The listing builds one solid part. Answer for the finished solid, in the listing's coordinates (mm). Face numbers are marked on the shaded views. A direction names the side the tool comes from. Round coordinates to 2 decimals unless told otherwise and drop trailing zeros. Write each loop counter-clockwise with the first axis right and the second up, starting at its lowest first coordinate (ties: lowest second). Pieces come first, ordered by that corner, then holes. Notation, with made-up numbers: (-15, 28) - (8, 28) arc R18 cw to (8, 42) - close; hole circle Ø3 at (44.5, 31). An arc over 180 degrees is marked (long way). Answer as CSV lines item,"result". Start each with the question number.
Item 1: For a pull along Y with two mould halves and no side action, classify the marked faces 1, 2, 3 and 4 as pulls with the +Y half, pulls with the -Y half, needs draft (parallel to the pull), parting line crosses it, or undercut.
Item 2: A cutting plane is placed at C-C on z = 132. Determine the outline of the cut face in (x, y), and give its area (3 significant figures).
Item 3: Which of the six approach directions +Z, -Z, +X, -X, +Y, -Y give full straight-line access (tool end or side, diameter ignored) to the marked faces 5 and 6?
Item 4: A cutting plane is placed at A-A on y = 10. Determine the outline of the cut face in (x, z), and give its area (3 significant figures).
Item 5: Straight lines are drawn through the part: line 1 along Z through (x, y) = (40, 74.5); line 2 along Z through (x, y) = (40, 86); line 3 along Y through (x, z) = (84, 42). For each, find the intervals that lie inside material, in ascending order. Write a range as [from, to].
Item 6: A cutting plane is placed at B-B on x = 44.5. Determine the outline of the cut face in (y, z), and give its area (3 significant figures).
Item 7: Flat-ended cylindrical pins translate along their axes: pin 1 (24 mm diameter, centred on x = 24, y = 32.5, fed in from -Z); pin 2 (8 mm diameter, centred on y = 63.5, z = 83.5, fed in from +X); pin 3 (8 mm diameter, centred on x = 49.5, z = 34, fed in from +Y); pin 4 (1.1 mm diameter, centred on x = 25.5, z = 81.5, fed in from +Y). Find the tip coordinate at first contact, or state that the pin passes through.
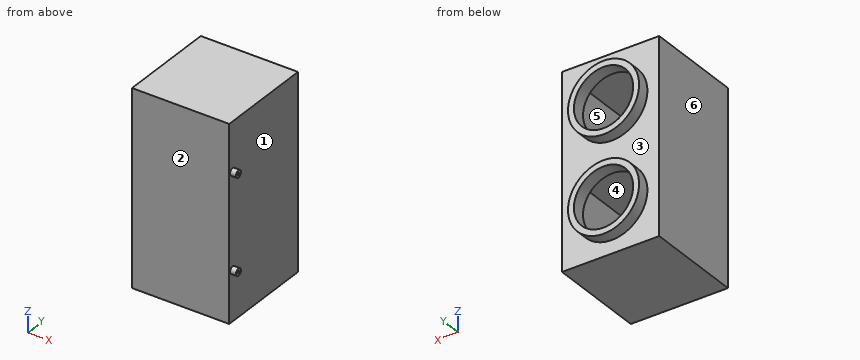
Autodesk Inventor part; units mm, degrees
ref_plane "YZ Plane" through (0, 0, 0) normal (1, 0, 0) x (0, 1, 0)
ref_plane "XZ Plane" through (0, 0, 0) normal (0, 1, 0) x (-1, 0, 0)
ref_plane "XY Plane" through (0, 0, 0) normal (0, 0, 1) x (1, 0, 0)
sketch "Sketch1" plane through (0, 0, 0) normal (0, 0, 1) x (1, 0, 0)
  line L0 (0, 0) -> (82, 0)
  line L1 (82, 0) -> (82, 82)
  line L2 (82, 82) -> (0, 82)
  line L3 (0, 82) -> (0, 0)
  dimension "d0" = 82
  dimension "d1" = 82
extrude "Extrusion1" add sketch "Sketch1" along normal blind 163
shell "Shell1" thickness 1 removed faces 1 at (54.6667, 82, 54.3333)
sketch "Sketch6" plane through (82, 0, 0) normal (1, 0, 0) x (0, 0, -1)
  circle A0 centre (-122, 4) radius 1
  circle A1 centre (-122, 4) radius 3
  line L0 (0, 0) -> (0, 82)
  line L1 (0, 0) -> (-163, 0)
  line L2 (-163, 0) -> (-163, 82)
  dimension "d18" = 2
  dimension "d19" = 2
  dimension "d21" = 4
  dimension "d50" = 41
extrude "Extrusion5" add sketch "Sketch6" along normal blind 5
thread "Thread1"
sketch "Sketch7" plane through (82, 4, 122) normal (1, 0, 0) x (0, 0, -1)
  circle A0 centre (0, 0) radius 1
  circle A1 centre (0, 0) radius 1
  point P0 (122, -4)
extrude "Extrusion6" cut sketch "Sketch7" against normal blind 5
sketch "Sketch8" plane through (0, 82, 0) normal (0, 1, 0) x (1, 0, 0)
  line L0 (0, 0) -> (0, -163)
  line L1 (82, 0) -> (82, -163)
  line L2 (0, 0) -> (82, 0)
  line L3 (82, 0) -> (82, -163)
  line L4 (82, -163) -> (0, -163)
  line L5 (0, -163) -> (0, 0)
  point P0 (0, -163)
extrude "Extrusion7" add sketch "Sketch8" along normal blind 1
sketch "Sketch9" plane through (0, 83, 0) normal (0, 1, 0) x (1, 0, 0)
  circle A0 centre (40, -122) radius 25
  circle A1 centre (40, -122) radius 30
  line L0 (0, 0) -> (0, -163)
  line L1 (0, -163) -> (82, -163)
  line L2 (1, -1) -> (1, -162)
  line L3 (1, -81.5) -> (81, -81.5)
  line L4 (81, -1) -> (81, -162)
  dimension "d30" = 50
  dimension "d31" = 40
  dimension "d32" = 41
  dimension "d33" = 5
extrude "Extrusion8" add sketch "Sketch9" along normal blind 10
sketch "Sketch10" plane through (40, 83, 122) normal (0, 1, 0) x (1, 0, 0)
  circle A0 centre (0, 0) radius 25
  point P0 (-40, 122)
extrude "Extrusion9" cut sketch "Sketch10" against normal blind 10
thread "Thread2"
sketch "Sketch12" plane through (1, 1, 1) normal (0, 1, 0) x (1, 0, 0)
  line L0 (0, 0) -> (0, -161)
  line L1 (0, -81) -> (80, -81)
  line L2 (80, -81) -> (80, -80)
  line L3 (80, -80) -> (0, -80)
  line L4 (0, -80) -> (0, -81)
  line L5 (80, 0) -> (80, -161)
  line L6 (0, -161) -> (80, -161)
  point P0 (-1, 1)
  point P1 (0, -80)
  dimension "d44" = 1
  dimension "d45" = 80
extrude "Extrusion11" add sketch "Sketch12" along normal blind 80 contours L3 L2 L1 L0
sketch "Sketch3" plane through (1, 82, 1) normal (0, 0, 1) x (1, 0, 0)
  line L0 (0, -81) -> (80, -81)
  line L1 (80, -81) -> (0, -78)
  line L2 (0, -78) -> (0, -81)
  point P0 (-1, -82)
  dimension "d5" = 3
extrude "Extrusion12" add sketch "Sketch3" along normal up to surface (161 mm away)
pattern_linear "Rectangular Pattern1" count 2 spacing 81 along (0, 0, -1) of "Extrusion8", "Extrusion9"
pattern_linear "Rectangular Pattern3" count 2 spacing 80 along (0, 0, -1) of "Extrusion5", "Extrusion6"
properties part number "BoxChem"
Geometry says:
1,face 1,"needs draft"
1,face 2,"pulls with the -Y half"
1,face 3,"pulls with the +Y half"
1,face 4,"undercut"
2,outline,"(0, 0) - (82, 0) - (82, 83) - (68.28, 83) - (68.28, 93) - (62.91, 93) - (62.91, 82) - (81, 82) - (81, 1) - (1, 4) - (1, 82) - (17.09, 82) - (17.09, 93) - (11.72, 93) - (11.72, 83) - (0, 83) - close"
2,area,"508 mm^2"
3,face 5,"none"
3,face 6,"+Z, -Z, -X, +Y, -Y"
4,outline,"(0, 0) - (82, 0) - (82, 163) - (0, 163) - close; hole (1, 1) - (81, 1) - (81, 81) - (1, 81) - close; hole (1, 82) - (81, 82) - (81, 162) - (1, 162) - close"
4,area,"566 mm^2"
5,line 1,"z = [0, 1], [81, 82], [162, 163]"
5,line 2,"z = [11, 16], [66, 71], [92, 97], [147, 152]"
5,line 3,"y = [1, 3], [5, 7]"
6,outline,"(0, 0) - (83, 0) - (83, 11.34) - (93, 11.34) - (93, 16.41) - (82, 16.41) - (82, 1) - (2.37, 1) - (2.37, 81) - (81, 81) - (81, 82) - (2.37, 82) - (2.37, 162) - (82, 162) - (82, 146.59) - (93, 146.59) - (93, 151.66) - (83, 151.66) - (83, 163) - (0, 163) - close; (82, 65.59) - (93, 65.59) - (93, 70.66) - (83, 70.66) - (83, 92.34) - (93, 92.34) - (93, 97.41) - (82, 97.41) - close"
6,area,"891 mm^2"
7,pin 1,"stops at z = 0"
7,pin 2,"stops at x = 82"
7,pin 3,"stops at y = 2.33"
7,pin 4,"stops at y = 83"
